Autodesk Inventor part; units mm, degrees
ref_plane "Work Plane1" through (-54.6393, -27.54, 0) normal (0, 0, 1) x (1, 0, 0)
ref_plane "YZ Plane" through (0, 0, 0) normal (1, 0, 0) x (0, 1, 0)
ref_plane "XZ Plane" through (0, 0, 0) normal (0, 1, 0) x (-1, 0, 0)
sketch "Sketch1" plane through (0, 0, 0) normal (0, 0, 1) x (1, 0, 0)
  line L0 (-13.6843, -5.4848) -> (-23.1843, -10.9697)
  line L1 (-23.1843, -10.9697) -> (-32.6843, -5.4848)
  line L2 (-32.6843, -5.4848) -> (-32.6843, 5.4848)
  line L3 (-32.6843, 5.4848) -> (-23.1843, 10.9697)
  line L4 (-23.1843, 10.9697) -> (-13.6843, 5.4848)
  line L5 (-13.6843, 5.4848) -> (-13.6843, -5.4848)
  circle A0 centre (13.3507, 17.0193) radius 2.54
  circle A1 centre (13.3507, -17.4028) radius 2.54
  circle A2 centre (13.3507, 0) radius 2.54
  circle A3 centre (-23.0489, 17.0193) radius 2.54
  circle A4 centre (-23.2, -17.4028) radius 2.54
  line L6 (-54.6393, -27.54) -> (18.4307, -27.54)
  line L7 (18.4307, -27.54) -> (18.4307, 27.54)
  line L8 (-54.6393, 27.54) -> (18.4307, 27.54)
  line L9 (-54.6393, -27.54) -> (-54.6393, 27.54)
  arc A5 (-23.1843, 23.0689) -> (-23.1843, 10.9697) centre (-23.0489, 17.0193) ccw
  line L10 (-23.1843, 10.9697) -> (-13.6843, 5.4848)
  line L11 (-13.6843, 5.4848) -> (-13.6843, -5.4848)
  line L12 (-13.6843, -5.4848) -> (-23.1843, -10.9697)
  line L13 (-23.1843, -23.6032) -> (-23.1843, -27.54)
  line L14 (-23.1843, 23.0689) -> (-23.1843, 27.54)
  line L15 (-23.1843, -27.54) -> (18.4307, -27.54)
  line L16 (18.4307, -27.54) -> (18.4307, 27.54)
  line L17 (18.4307, 27.54) -> (-23.1843, 27.54)
  arc A6 (-23.1843, -10.9697) -> (-23.1843, -23.6032) centre (-22.7708, -17.2864) ccw
  point P0 (0, 0)
extrude "Extrusion1" add sketch "Sketch1" along normal blind 5.08 contours L5 L4 A5 L14 L8 L7 L6 L13 A6 L0
chamfer "Chamfer1" distance 1.5875 angle 45 4 edges at (-23.1843, -27.54, 2.54) (-23.1843, 27.54, 2.54) (-23.1843, 23.0689, 2.54) (-23.1843, -23.6032, 2.54)
sketch "Sketch2" plane through (18.4307, -27.54, 0) normal (1, 0, 0) x (0, 0, -1)
  line L0 (25.4, 55.08) -> (25.4, 29.5535)
  line L1 (25.4, 29.5535) -> (38.1, 29.5535)
  point P0 (0, 27.54)
  dimension "d5" = 12.7
sketch "Sketch3" plane through (0, 0, 5.08) normal (0, 0, 1) x (1, 0, 0)
  line L0 (-23.1843, 25.9525) -> (-21.5968, 27.54)
  line L1 (-23.1843, 25.9525) -> (-23.1843, 24.6564)
  line L2 (-24.753, 22.8255) -> (-23.1843, 24.6564)
  arc A0 (-24.753, 22.8255) -> (-23.1843, 10.9697) centre (-23.0489, 17.0193) ccw
  line L3 (-23.1843, 10.9697) -> (-13.6843, 5.4848)
  line L4 (-13.6843, 5.4848) -> (-13.6843, -5.4848)
  line L5 (-13.6843, -5.4848) -> (-23.1843, -10.9697)
  arc A1 (-23.1843, -10.9697) -> (-24.7429, -23.3017) centre (-22.7708, -17.2864) ccw
  line L6 (-23.1843, -25.1907) -> (-24.7429, -23.3017)
  line L7 (-23.1843, -25.1907) -> (-23.1843, -25.9525)
  line L8 (-21.5968, -27.54) -> (-23.1843, -25.9525)
  line L9 (-21.5968, -27.54) -> (18.4307, -27.54)
  line L10 (18.4307, -27.54) -> (18.4307, 27.54)
  line L11 (18.4307, 27.54) -> (-21.5968, 27.54)
  circle A2 centre (-23.2, -17.4028) radius 2.54
  circle A3 centre (-23.0489, 17.0193) radius 2.54
  circle A4 centre (13.3507, 0) radius 2.54
  circle A5 centre (13.3507, -17.4028) radius 2.54
  circle A6 centre (13.3507, 17.0193) radius 2.54
  line L12 (18.4307, -17.4028) -> (24.9307, -17.4028)
  line L13 (24.9307, -17.4028) -> (30.9307, -17.4028)
  arc A7 (30.9307, -11.4028) -> (30.9307, -23.4028) centre (30.9307, -17.4028) ccw
  line L14 (30.9307, -23.4028) -> (30.9307, -27.54)
  line L15 (30.9307, -27.54) -> (18.4307, -27.54)
  line L16 (18.4307, 0) -> (20.9229, 0)
  line L17 (18.4307, 17.4028) -> (24.9307, 17.4028)
  line L18 (24.9307, 17.4028) -> (30.9307, 17.4028)
  arc A8 (30.9307, 23.4028) -> (30.9307, 11.4028) centre (30.9307, 17.4028) ccw
  line L19 (30.9307, 23.4028) -> (30.9307, 27.54)
  line L20 (30.9307, 27.54) -> (18.4307, 27.54)
  line L21 (30.9307, -11.4028) -> (30.9307, 11.4028)
  point P0 (0, 0)
  dimension "d6" = 6.5
  dimension "d7" = 6
  dimension "d8" = 6
ref_plane "Work Plane1" through (-54.6393, -27.54, 0) normal (0, 0, 1) x (1, 0, 0)
extrude "Extrusion2" add sketch "Sketch3" against normal up to surface (5.08 mm away) contours L20 L19 A8 L17 L10 | L17 A8 L21 A7 L12 L10 | L12 A7 L14 L15 L10
sketch "Sketch4" plane through (0, 0, 5.08) normal (0, 0, 1) x (1, 0, 0)
  line L0 (-23.1843, 25.9525) -> (-21.5968, 27.54)
  line L1 (-23.1843, 25.9525) -> (-23.1843, 24.6564)
  line L2 (-24.753, 22.8255) -> (-23.1843, 24.6564)
  arc A0 (-24.753, 22.8255) -> (-23.1843, 10.9697) centre (-23.0489, 17.0193) ccw
  line L3 (-23.1843, 10.9697) -> (-13.6843, 5.4848)
  line L4 (-13.6843, 5.4848) -> (-13.6843, -5.4848)
  line L5 (-13.6843, -5.4848) -> (-23.1843, -10.9697)
  arc A1 (-23.1843, -10.9697) -> (-24.7429, -23.3017) centre (-22.7708, -17.2864) ccw
  line L6 (-23.1843, -25.1907) -> (-24.7429, -23.3017)
  line L7 (-23.1843, -25.1907) -> (-23.1843, -25.9525)
  line L8 (-21.5968, -27.54) -> (-23.1843, -25.9525)
  line L9 (-21.5968, -27.54) -> (30.9307, -27.54)
  line L10 (30.9307, -27.54) -> (30.9307, -23.4028)
  arc A2 (30.9307, -11.4028) -> (30.9307, -23.4028) centre (30.9307, -17.4028) ccw
  line L11 (30.9307, -11.4028) -> (30.9307, 11.4028)
  arc A3 (30.9307, 23.4028) -> (30.9307, 11.4028) centre (30.9307, 17.4028) ccw
  line L12 (30.9307, 23.4028) -> (30.9307, 27.54)
  line L13 (30.9307, 27.54) -> (-21.5968, 27.54)
  circle A4 centre (-23.2, -17.4028) radius 2.54
  circle A5 centre (-23.0489, 17.0193) radius 2.54
  circle A6 centre (13.3507, 0) radius 2.54
  circle A7 centre (13.3507, -17.4028) radius 2.54
  circle A8 centre (13.3507, 17.0193) radius 2.54
  line L14 (30.9307, -23.4028) -> (30.9307, -27.54)
  arc A9 (30.9307, -9.4028) -> (30.9307, -25.4028) centre (30.9307, -17.4028) ccw
  arc A10 (30.9307, 23.4028) -> (30.9307, 11.4028) centre (30.9307, 17.4028) ccw
  line L15 (30.9307, -11.4028) -> (30.9307, 11.4028)
  arc A11 (30.9307, 25.4028) -> (30.9307, 9.4028) centre (30.9307, 17.4028) ccw
  line L16 (-21.5968, -27.54) -> (30.9307, -27.54)
  line L17 (20.0107, -27.54) -> (20.0107, 27.54)
  line L18 (30.9307, 27.54) -> (-21.5968, 27.54)
  line L19 (20.0107, -26.7462) -> (20.0107, -27.54)
  line L20 (-21.5968, -27.54) -> (30.9307, -27.54)
  line L21 (20.0107, -27.54) -> (30.9307, -27.54)
  line L22 (30.9307, -27.54) -> (30.9307, -23.4028)
  line L23 (30.9307, -25.4028) -> (30.9307, -27.54)
  line L24 (30.9307, -9.4028) -> (30.9307, 9.4028)
  line L25 (20.0107, 27.54) -> (30.9307, 27.54)
  line L26 (30.9307, 27.54) -> (30.9307, 25.4028)
  line L27 (30.9307, 23.4028) -> (30.9307, 27.54)
  point P0 (0, 0)
  dimension "d11" = 8
  dimension "d12" = 8
extrude "Extrusion3" add sketch "Sketch4" along normal blind 4 contours L13 L12 A11 L11 A9 L10 L9 L17
sketch "Sketch5" plane through (-21.5968, -27.54, 0) normal (0, -1, 0) x (1, 0, 0)
  point P0 (21.5968, 0)
sketch "Sketch6" plane through (-21.5968, -27.54, 0) normal (0, -1, 0) x (1, 0, 0)
  line L0 (0, 0) -> (0, 5.08)
  line L1 (0, 0) -> (52.5275, 0)
  line L2 (52.5275, 0) -> (52.5275, 9.08)
  line L3 (41.6075, 9.08) -> (52.5275, 9.08)
  line L4 (41.6075, 5.08) -> (41.6075, 9.08)
  line L5 (0, 5.08) -> (41.6075, 5.08)
  line L6 (41.6075, 5.08) -> (41.6075, 9.08)
  line L7 (41.6075, 9.08) -> (30.9206, 5.08)
  line L8 (0, 5.08) -> (41.6075, 5.08)
  point P0 (21.5968, 0)
extrude "Extrusion4" add sketch "Sketch6" against normal blind 4 contours L7 L4 L5
sketch "Sketch7" plane through (-21.5968, 27.54, 5.08) normal (0, 1, 0) x (1, 0, 0)
  line L0 (41.6075, 0) -> (41.6075, -4)
  line L1 (30.9206, 0) -> (41.6075, 0)
  line L2 (30.9206, 0) -> (41.6075, -4)
  point P0 (21.5968, 5.08)
extrude "Extrusion5" add sketch "Sketch7" against normal blind 4
sketch "Sketch8" plane through (0, 0, 9.08) normal (0, 0, 1) x (1, 0, 0)
  line L0 (30.9307, -27.54) -> (30.9307, -25.4028)
  arc A0 (30.9307, -9.4028) -> (30.9307, -25.4028) centre (30.9307, -17.4028) ccw
  line L1 (30.9307, -9.4028) -> (30.9307, 9.4028)
  arc A1 (30.9307, 25.4028) -> (30.9307, 9.4028) centre (30.9307, 17.4028) ccw
  line L2 (30.9307, 25.4028) -> (30.9307, 27.54)
  line L3 (30.9307, 27.54) -> (20.0107, 27.54)
  line L4 (20.0107, 27.54) -> (20.0107, 23.54)
  line L5 (20.0107, 23.54) -> (20.0107, -23.54)
  line L6 (20.0107, -23.54) -> (20.0107, -27.54)
  line L7 (20.0107, -27.54) -> (30.9307, -27.54)
  line L8 (20.0107, 27.54) -> (30.9307, 27.54)
  line L9 (30.9307, 27.54) -> (30.9307, 37.7)
  line L10 (30.9307, 37.7) -> (20.0107, 37.7)
  line L11 (20.0107, 37.7) -> (20.0107, 27.54)
  line L12 (20.0107, -27.54) -> (30.9307, -27.54)
  line L13 (20.0107, -27.54) -> (30.9307, -27.54)
  line L14 (30.9307, -27.54) -> (30.9307, -37.7)
  line L15 (30.9307, -37.7) -> (20.0107, -37.7)
  line L16 (20.0107, -37.7) -> (20.0107, -27.54)
  point P0 (0, 0)
  dimension "d19" = 10.16
  dimension "d20" = 10.16
extrude "Extrusion6" add sketch "Sketch8" against normal up to surface (9.08 mm away) contours L14 L15 L16 L7 | L11 L10 L9 L3
sketch "Sketch9" plane through (30.9307, -23.4028, 5.08) normal (1, 0, 0) x (0, 0, -1)
  line L0 (5.08, 50.9428) -> (5.08, 61.1028)
  line L1 (-4, 50.9428) -> (5.08, 50.9428)
  line L2 (-4, 61.1028) -> (-4, 50.9428)
  line L3 (-4, 61.1028) -> (5.08, 61.1028)
  line L4 (5.08, -14.2972) -> (5.08, -4.1372)
  line L5 (-4, -14.2972) -> (5.08, -14.2972)
  line L6 (-4, -4.1372) -> (-4, -14.2972)
  line L7 (5.08, -4.1372) -> (-4, -4.1372)
  circle A0 centre (0.54, -9.2172) radius 1.5
  circle A1 centre (0.54, 56.0228) radius 1.5
  point P0 (5.08, 23.4028)
  dimension "d23" = 3
  dimension "d24" = 3
extrude "Extrusion7" cut sketch "Sketch9" against normal blind 18.2875 contours A0 | A1
sketch "Sketch10" plane through (30.9307, -11.4028, 0) normal (1, 0, 0) x (0, 0, -1)
  line L0 (-12.4469, -33.6461) -> (5.8759, -33.6461)
  line L1 (5.8759, -33.6461) -> (5.8759, 55.3145)
  line L2 (5.8759, 55.3145) -> (-12.4469, 55.3145)
  line L3 (-12.4469, 55.3145) -> (-12.4469, -33.6461)
  point P0 (0, 11.4028)
extrude "Extrusion8" cut sketch "Sketch10" against normal blind 0.5
properties part number "Hotend mount"
Could you check a few things on this model? Use its own coordinates, in mm. A direction names the side the tool comes from. Round coordinates to 2 decimals unless told otherwise and drop trailing zeros. Order: outer loops, then holes, each group sorted by start corner. A loop starts at its lowest first (then second) coordinate and runs counter-clockwise, first axis right, second up.
Q1. Which directions (+Z, -Z, +X, -X, +Y, -Y) give clear straight access to the entire face, cutting with the end or side of a thin tool? Please do faces 1 (the face through (-1, 27.54, 2)), 2 (the face through (17, -23.54, 6)), 3 (the face through (-18.501, 8.266, 2.504)).
Geometry says:
face 1: +Z, -Z, -X, +Y
face 2: +Z, -X
face 3: +Z, -Z, -X
Q2. Imagine slicing it at B-B, the plane y = 0. List the corners of the cut face in (x, z) for me, then the cut area to 3 significant figures.
Geometry says:
outline: (-13.68, 0) - (10.81, 0) - (10.81, 5.08) - (-13.68, 5.08) - close; (15.89, 0) - (30.43, 0) - (30.43, 9.08) - (20.01, 9.08) - (20.01, 5.08) - (15.89, 5.08) - close
area: 240 mm2
Q3. Please list where these lines run through material, in increasing order: probe 1 along Y at (x, z) = (24.5, 4.54); probe 2 along Y at (x, z) = (-22.5, 3); probe 3 along Y at (x, z) = (28, 4.54).
Geometry says:
probe 1: y = -37.7 to -34.12, -31.12 to 31.12, 34.12 to 37.7
probe 2: y = -26.64 to -19.84, -14.96 to -10.57, 10.57 to 14.54, 19.5 to 26.64
probe 3: y = -37.7 to -34.12, -31.12 to -22.64, -12.17 to 12.17, 22.64 to 31.12, 34.12 to 37.7
Q4. I'm going to push flat-ended pins straight in: P1, Ø3.5, axis at y = -32.62, z = 4.54, coming from the +X side; P2, Ø1.2, axis at x = 14.5, z = 7.5, coming from the +Y side; P3, Ø3, axis at x = 13.5, z = 7.5, coming from the -Y side; P4, Ø3, axis at y = -17, z = 7.5, coming from the +X side. Where does each tip first touch, or does it pass through?
Geometry says:
P1: stops at x = 30.43
P2: stops at y = 27.54
P3: stops at y = -27.54
P4: stops at x = 23.16
Q5. Imagine slicing it at C-C, the plane z = 1.25. List the corners of the cut face in (x, y) for me.
Geometry says:
outline: (-24.75, 22.83) arc R6.05 ccw to (-23.18, 10.97) - (-13.68, 5.48) - (-13.68, -5.48) - (-23.18, -10.97) arc R6.33 ccw to (-24.74, -23.3) - (-23.18, -25.19) - (-23.18, -25.95) - (-21.6, -27.54) - (20.01, -27.54) - (20.01, -37.7) - (30.43, -37.7) - (30.43, -23.38) arc R6 cw to (30.43, -11.42) - (30.43, 11.42) arc R6 cw to (30.43, 23.38) - (30.43, 37.7) - (20.01, 37.7) - (20.01, 27.54) - (-21.6, 27.54) - (-23.18, 25.95) - (-23.18, 24.66) - close; hole circle Ø5.08 at (-23.2, -17.4); hole circle Ø5.08 at (-23.05, 17.02); hole circle Ø5.08 at (13.35, -17.4); hole circle Ø5.08 at (13.35, 0); hole circle Ø5.08 at (13.35, 17.02)
Q6. Imagine slicing it at D-D, the plane x = -17.5. List the corners of the cut face in (y, z) for me.
Geometry says:
outline: (-27.54, 0) - (-7.69, 0) - (-7.69, 5.08) - (-27.54, 5.08) - close; (7.69, 0) - (27.54, 0) - (27.54, 5.08) - (7.69, 5.08) - close
Q7. Thinking about a two-plate mould opening in X: for faces 4 (the face through (11.48, 15.3, 2.5)), 5 (the face through (-20.626, 16.256, 2.504)), 6 (the face through (22.932, 17.234, 7.052)), 7 (the face through (14.59, 25.57, 7.05)), which applies, released by +X, released by -X, zero draft, split by the parting line, or undercut?
Geometry says:
face 4: undercut
face 5: undercut
face 6: released by +X
face 7: released by -X
Q8. Imagine slicing it at A-A, the plane x = 27. List the corners of the cut face in (y, z) for me, then the cut area to 3 significant figures.
Geometry says:
outline: (-37.7, 0) - (-21.94, 0) - (-21.94, 5.08) - (-24.37, 5.08) - (-24.37, 9.08) - (-37.7, 9.08) - close; (-12.87, 0) - (12.87, 0) - (12.87, 5.08) - (10.44, 5.08) - (10.44, 9.08) - (-10.44, 9.08) - (-10.44, 5.08) - (-12.87, 5.08) - close; (21.94, 0) - (37.7, 0) - (37.7, 9.08) - (24.37, 9.08) - (24.37, 5.08) - (21.94, 5.08) - close; hole circle Ø3 at (-32.62, 4.54); hole circle Ø3 at (32.62, 4.54)
area: 467 mm2
